```python
from build123d import *

# Parameters (mm, degrees)
PATTERN_CIRCULAR_1_COUNT           = 4
CHAMFER_1_SIZE                     = 1
CHAMFER_2_SIZE                     = 1
MM_1_D                             = 6
MM_1_DEPTH                         = 6
MM_1_TIP                           = 1.802581857
SKETCH_12_W                        = 2.1
SKETCH_12_H                        = 41.012198951
HOLE_WIZARD_M5_2_AT_2_COUNT        = 2
HOLE_WIZARD_M5_2_AT_2_PITCH        = 8
PATTERN_CIRCULAR_3_COUNT           = 4
PATTERN_CIRCULAR_3_COPY_1_SKETCH_W = 2.1
PATTERN_CIRCULAR_3_COPY_1_SKETCH_H = 41.012198951
PATTERN_CIRCULAR_3_COPY_2_SKETCH_W = 2.1
PATTERN_CIRCULAR_3_COPY_2_SKETCH_H = 41.012198951
PATTERN_CIRCULAR_3_COPY_3_SKETCH_W = 2.1
PATTERN_CIRCULAR_3_COPY_3_SKETCH_H = 41.012198951


with BuildPart() as part:
    # 草图1 → 旋转1 (revolve)
    with BuildSketch(Plane(origin=(0, 0, 0), x_dir=(0, 0, -1), z_dir=(1, 0, 0)), mode=Mode.PRIVATE) as revolve_1_sk:
        Polygon((64, 29), (64, 10), (40, 10), (40, 17.5), (0, 17.5), (0, 29), align=None)
    revolve(revolve_1_sk.sketch.rotate(Axis((0, 0, 74.600938967), (0, 0, -1)), 90), axis=Axis((0, 0, 74.600938967), (0, 0, -1)))

    # 草图5 → M5 螺纹孔1 (revolve, cut)
    with BuildSketch(Plane(origin=(15.909902577, 15.909902577, 0), x_dir=(0, -1, 0), z_dir=(1, 0, 0))):
        Polygon((0, 0), (0, 15.2618073), (2.1, 14), (2.1, 0), align=None)
    hole_wizard_m5_1 = revolve(axis=Axis((15.909902577, 15.909902577, 6.35), (0, 0, -1)), mode=Mode.SUBTRACT)

    # 阵列(圆周)1: M5 螺纹孔1 ×4 about axis
    pattern_circular_1_axis = Axis((0, 0, 0), (0, 0, 1))
    for i in range(1, PATTERN_CIRCULAR_1_COUNT):
        add(hole_wizard_m5_1.rotate(pattern_circular_1_axis, i * 360 / PATTERN_CIRCULAR_1_COUNT), mode=Mode.SUBTRACT)

    # 倒角1
    chamfer_1_edges = [part.edges().sort_by_distance(p)[0] for p in [
        (-29, 0, 0),
        (-29, 0, -64),
    ]]
    chamfer(chamfer_1_edges, length=CHAMFER_1_SIZE)

    # 倒角2
    chamfer_2_edges = [part.edges().sort_by_distance(p)[0] for p in [
        (-10, 0, -64),
        (-10, 0, -40),
        (-17.5, 0, 0),
    ]]
    chamfer(chamfer_2_edges, length=CHAMFER_2_SIZE)

    # 大小mm 暗销孔1
    with Locations(Plane.XY):
        with Locations((0, -22.5), (-22.5, 0), (0, 22.5), (22.5, 0)):
            Hole(MM_1_D / 2, depth=MM_1_DEPTH)
            with Locations((0, 0, -(MM_1_DEPTH + MM_1_TIP / 2))):  # 118° drill point
                Cone(0, MM_1_D / 2, MM_1_TIP, mode=Mode.SUBTRACT)

    # 草图12 → M5 螺纹孔2 (revolve, cut)
    with BuildSketch(Plane(origin=(-2.992e-06, 2.992e-06, -48), x_dir=(-0.4082482226009898, -0.4082483243953038, 0.8164965978934386), z_dir=(0.5773503171759193, 0.5773502451964775, 0.5773502451964775))):
        with Locations((1.05, 20.506099476)):
            Rectangle(SKETCH_12_W, SKETCH_12_H)
    hole_wizard_m5_2 = revolve(axis=Axis((-4.490131053, 4.490131053, -47.99999944), (0.7071067811865461, -0.7071067811865434, -8.815645872088268e-08)), mode=Mode.SUBTRACT)

    # M5 螺纹孔2 at 2: M5 螺纹孔2 ×2
    with Locations(*[(0, 0, -i * HOLE_WIZARD_M5_2_AT_2_PITCH) for i in range(1, HOLE_WIZARD_M5_2_AT_2_COUNT)]):
        add(hole_wizard_m5_2, mode=Mode.SUBTRACT)

    # 阵列(圆周)3: M5 螺纹孔2 ×4 about axis
    pattern_circular_3_axis = Axis((0, 0, -63), (0, 0, -1))
    for i in range(1, PATTERN_CIRCULAR_3_COUNT):
        add(hole_wizard_m5_2.rotate(pattern_circular_3_axis, i * 360 / PATTERN_CIRCULAR_3_COUNT), mode=Mode.SUBTRACT)

    # 阵列(圆周)3 copy 1 sketch → 阵列(圆周)3 copy 1 (revolve, cut)
    with BuildSketch(Plane(origin=(3.491e-06, 3.491e-06, -56), x_dir=(-0.4082483243953038, 0.4082482226009898, 0.8164965978934386), z_dir=(0.5773502451964775, -0.5773503171759193, 0.5773502451964775))):
        with Locations((1.05, 20.506099476)):
            Rectangle(PATTERN_CIRCULAR_3_COPY_1_SKETCH_W, PATTERN_CIRCULAR_3_COPY_1_SKETCH_H)
    revolve(axis=Axis((4.490131551, 4.490131551, -55.99999944), (-0.7071067811865434, -0.7071067811865461, -8.815645872088268e-08)), mode=Mode.SUBTRACT)

    # 阵列(圆周)3 copy 2 sketch → 阵列(圆周)3 copy 2 (revolve, cut)
    with BuildSketch(Plane(origin=(3.491e-06, -3.491e-06, -56), x_dir=(0.40824822260098975, 0.40824832439530384, 0.8164965978934386), z_dir=(-0.5773503171759192, -0.5773502451964776, 0.5773502451964775))):
        with Locations((1.05, 20.506099476)):
            Rectangle(PATTERN_CIRCULAR_3_COPY_2_SKETCH_W, PATTERN_CIRCULAR_3_COPY_2_SKETCH_H)
    revolve(axis=Axis((4.490131551, -4.490131551, -55.99999944), (-0.7071067811865462, 0.7071067811865432, -8.815645872088268e-08)), mode=Mode.SUBTRACT)

    # 阵列(圆周)3 copy 3 sketch → 阵列(圆周)3 copy 3 (revolve, cut)
    with BuildSketch(Plane(origin=(-3.491e-06, -3.491e-06, -56), x_dir=(0.40824832439530384, -0.40824822260098975, 0.8164965978934386), z_dir=(-0.5773502451964776, 0.5773503171759192, 0.5773502451964775))):
        with Locations((1.05, 20.506099476)):
            Rectangle(PATTERN_CIRCULAR_3_COPY_3_SKETCH_W, PATTERN_CIRCULAR_3_COPY_3_SKETCH_H)
    revolve(axis=Axis((-4.490131551, -4.490131551, -55.99999944), (0.7071067811865432, 0.7071067811865462, -8.815645872088268e-08)), mode=Mode.SUBTRACT)


solid = part.part
```
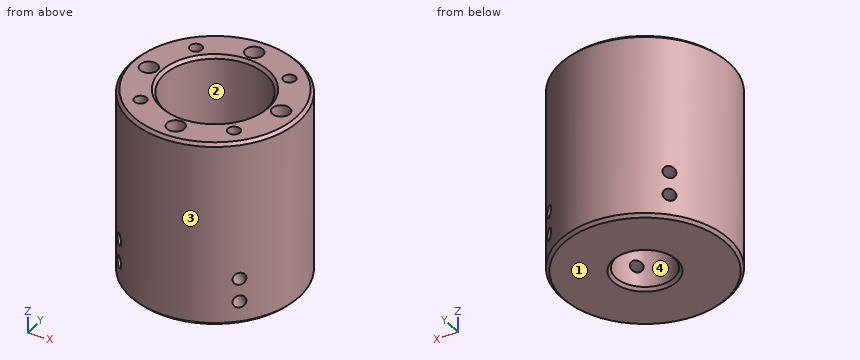
CAD build for the part. Positions are in the model's coordinates, mm. Face numbers are marked on the shaded views. Coordinates: 2 decimals unless noted, no trailing zeros. Write each loop counter-clockwise with the first axis right and the second up, starting at its lowest first coordinate (ties: lowest second). Pieces come first, ordered by that corner, then holes.
(1) Cut at B-B, the plane y = -12. Count the separate pieces of the cut face and the enclosed holes in it, and give its area (3 significant figures).
(2) Two-plate mould, pull along X, no slides. Class the marked faces 1, 2, 3 and 4: +X half, -X half, draft (parallel to the pull), parting line (faces both ways), or undercut.
(3) Cut at D-D, the plane z = -53. List the corners of the cut face in (x, y).
(4) Flat gauge pins, fed straight in: pin 1 (1 mm diameter, centred on y = 5, z = -11, fed in from -X); pin 2 (5 mm diameter, centred on x = 0, y = 22.5, fed in from +Z); pin 3 (5 mm diameter, centred on y = 13, z = -13, fed in from -X); pin 4 (2 mm diameter, centred on x = -11.5, y = 18.5, fed in from +Z). Where does each tip first touch, or does it go through?
(5) Drill centre lines: probe 1 along Y at (x, z) = (0, -3); probe 2 along Y at (x, z) = (0, -11.5); probe 3 along Y at (x, z) = (25.5, -21). Where is each one in solid material? Low to high.
(6) Cut at A-A, the plane z = -21.5. List the corners of the cut face in (x, y), and give its area (3 significant figures).
Geometry says:
1. separate pieces: 1
1. enclosed holes: 4
1. area: 2,280 mm2
2. face 1: draft
2. face 2: undercut
2. face 3: parting line
2. face 4: undercut
3. outline: circle Ø58 at (0, 0); hole circle Ø20 at (0, 0)
4. pin 1: stops at x = -28.65
4. pin 2: stops at z = -6.3
4. pin 3: stops at x = -27.03
4. pin 4: stops at z = 0
5. probe 1: y = -29 to -25.5, -19.5 to -17.5, 17.5 to 19.5, 25.5 to 29
5. probe 2: y = -29 to -17.5, 17.5 to 29
5. probe 3: y = -13.81 to 13.81
6. outline: circle Ø58 at (0, 0); hole circle Ø35 at (0, 0)
6. area: 1,680 mm2
